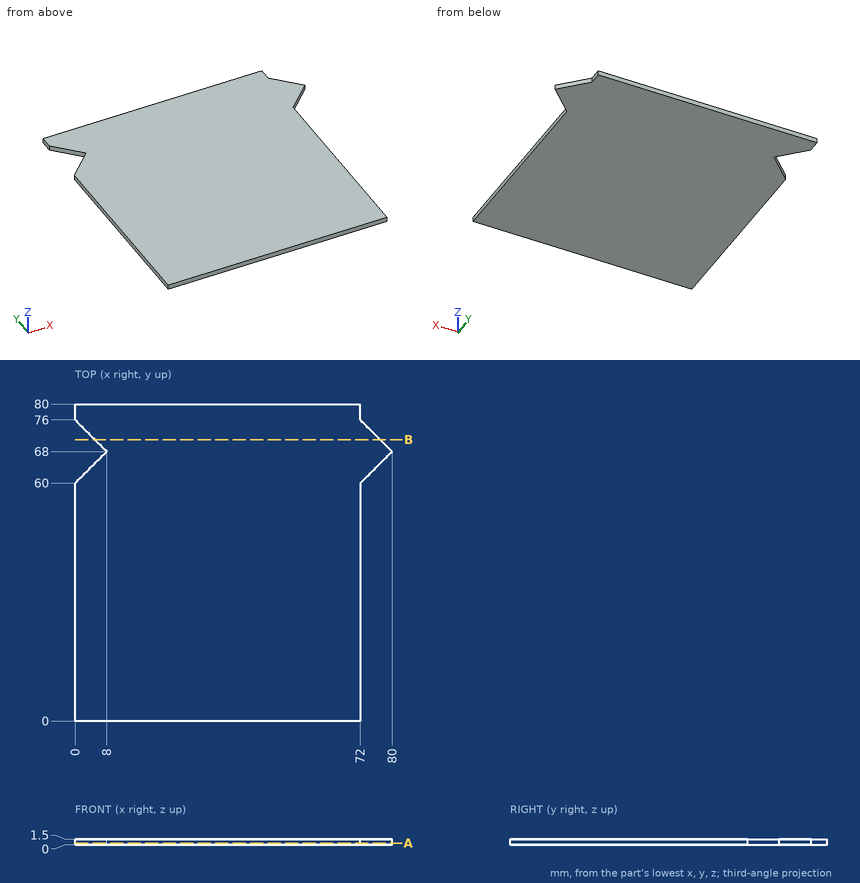
The drawing under review shows one solid part. Ordinate dimensions are in mm from its lowest x, y, z. Coordinates: 2 decimals unless noted, no trailing zeros. Write each loop counter-clockwise with the first axis right and the second up, starting at its lowest first coordinate (ties: lowest second). Pieces come first, ordered by that corner, then holes. Notation, with made-up numbers: M -4.5,62 L 44.5,62 A24 cw 44.5,73 Z; hole C 54,0 d5. An arc over 180 degrees is marked long. Put each result on its own line as item: value.
1) Clearance check with a flat-ended pin moving along its axis: pin 1 Ø2 at (x, y) = (42.5, 21.5) entering from -Z. State where the tip first meets the part, or that it passes through.
Computed:
pin 1: stops at z = 0
2) Wall thickness on probe 1 along X at (y, z) = (76.5, 0.2); probe 2 along X at (y, z) = (74, 0.3); probe 3 along Y at (x, z) = (75.5, 0.8): over which ranges is each line inside the solid? List them lowest first. Write a range as [from, to].
Computed:
probe 1: x = [0, 72]
probe 2: x = [2, 74]
probe 3: y = [63.5, 72.5]
3) Add section A-A on z = 0.45. Give the boundary of the cut face in (x, y), then the cut area to 3 significant figures.
Computed:
outline: M 0,0 L 72,0 L 72,60 L 80,68 L 72,76 L 72,80 L 0,80 L 0,76 L 8,68 L 0,60 Z
area: 5,760 mm2
4) Add section B-B on y = 71. Give the boundary of the cut face in (x, z).
Computed:
outline: M 5,0 L 77,0 L 77,1.5 L 5,1.5 Z
